Could you check a few things on this drawing? It's one solid part, dimensions in mm from its lowest x, y, z. Round coordinates to 2 decimals unless told otherwise and drop trailing zeros. Write each loop counter-clockwise with the first axis right and the second up, starting at its lowest first coordinate (ties: lowest second). Pieces come first, ordered by that corner, then holes. Notation, with made-up numbers: (16.5, 58) -> (28.5, 58) arc R13 ccw to (28.5, 64) -> close; hole circle Ø10 at (68, 81.5). An arc over 180 degrees is marked (long way). Put each result on its own line as item: value. Start each with the question number.
1) I want a section at B-B, the plane x = 33. List the corners of the cut face in (y, z) for me, then the cut area to 3 significant figures.
2) I want a section at A-A, the plane y = 1.75. List the corners of the cut face in (x, z) for me, then the cut area to 3 significant figures.
3) We'd pull the mould along Z, two halves only. Please class the marked faces 1, 2 and 3: released by +Z, released by -Z, zero draft, split by the parting line, or undercut.
4) If I drill on line 1 along X through (y, z) = (11.25, 31.5); line 2 along X through (y, z) = (2.5, 30), over which ranges is the centre line in solid material (lowest first)? Write a range as [from, to].
5) Will these pins go through, and if not, where does the flat tip stop? P1, Ø5, axis at x = 32, z = 19, coming from the -Y side; P2, Ø3, axis at x = 34, z = 31.14, coming from the -Y side.
6) I want a section at C-C, the plane z = 35.5. List the corners of the cut face in (x, y) for me (1 decimal).
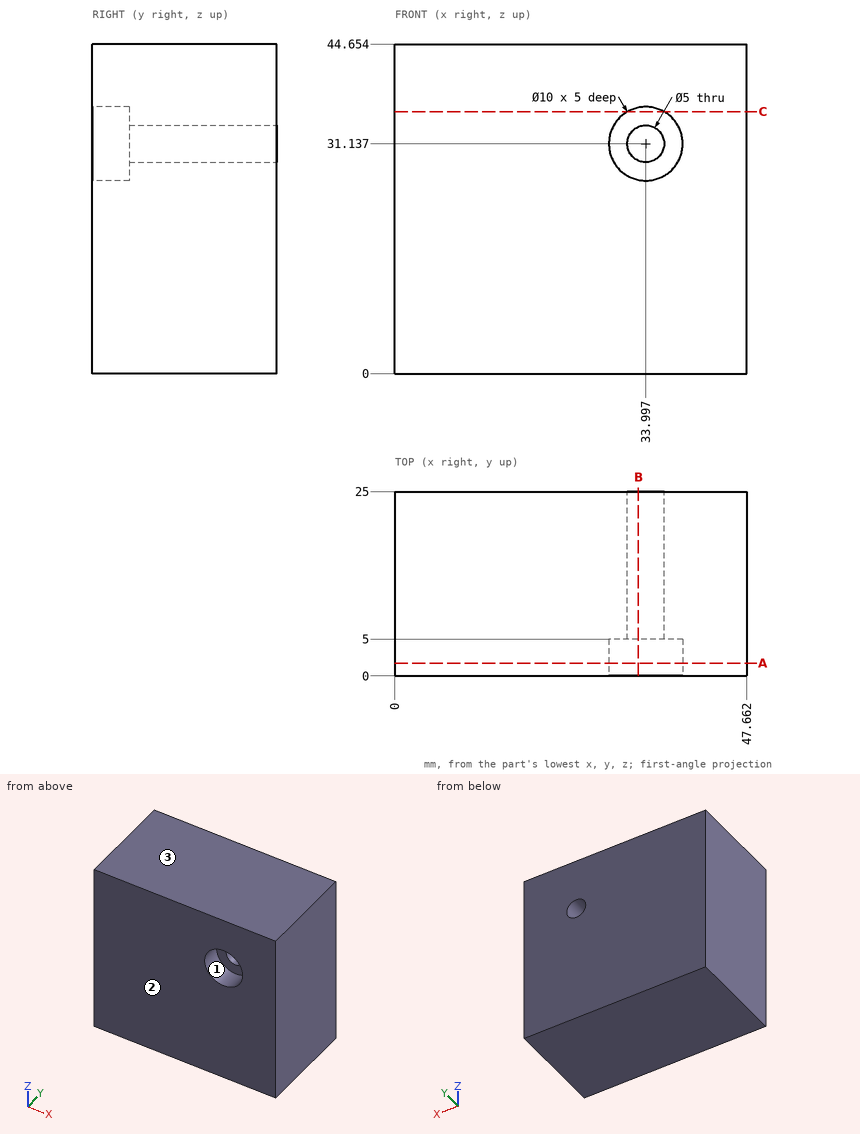
Findings:
1. outline: (0, 0) -> (25, 0) -> (25, 28.84) -> (5, 28.84) -> (5, 26.24) -> (0, 26.24) -> close; (0, 36.04) -> (5, 36.04) -> (5, 33.43) -> (25, 33.43) -> (25, 44.65) -> (0, 44.65) -> close
1. area: 976 mm2
2. outline: (0, 0) -> (47.66, 0) -> (47.66, 44.65) -> (0, 44.65) -> close; hole circle Ø10 at (34, 31.14)
2. area: 2,050 mm2
3. face 1: undercut
3. face 2: zero draft
3. face 3: released by +Z
4. line 1: x = [0, 31.52], [36.47, 47.66]
4. line 2: x = [0, 29.13], [38.87, 47.66]
5. P1: stops at y = 0
5. P2: passes through
6. outline: (0, 0) -> (31.6, 0) -> (31.6, 5) -> (36.4, 5) -> (36.4, 0) -> (47.7, 0) -> (47.7, 25) -> (0, 25) -> close
